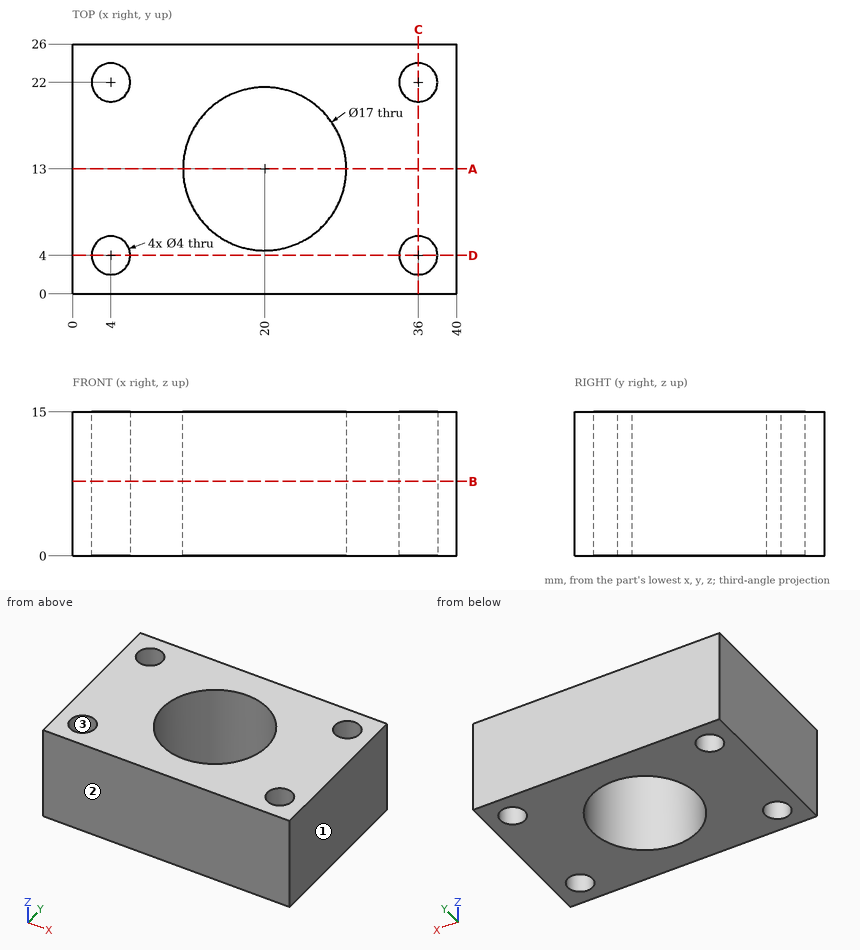
For this review, use the dimensioned drawing (mm, ordinates from the lowest corner) and the shaded views. Give positions to 0.01 mm unless a question says otherwise; leave off trailing zeros. Order: outer loops, then holes, each group sorted by start corner. A loop starts at its lowest first (then second) coordinate and runs counter-clockwise, first axis right, second up. Notation, with made-up numbers: (13.5, 28) - (58.5, 28) arc R21 cw to (58.5, 37) - close; hole circle Ø9 at (26.5, -28.5). An arc over 180 degrees is marked (long way). Write item = value, one per line. Start each with the question number.
Q1. We need section B-B on z = 7.75. State the section outline as (x, y) points, plus the area to 3 significant figures.
Q2. Mouldability with a two-part tool opening along X and no side actions: class the marked faces 1, 2 and 3 as released by +X, released by -X, zero draft, split by the parting line, or undercut.
Q3. We need section C-C on x = 36. State the section outline as (y, z) points.
Q4. To check wall thickness, follow L1, parallel to Y at x = 4, z = 5.25; L2, parallel to X at y = 2.25, z = 14.25; L3, parallel to Y at x = 37.5, z = 10.5. State the ranges of each line that lie inside material, in increasing order. Write a range as from..to.
Q5. We need section A-A on y = 13. State the section outline as (x, z) points.
Q6. Clearance check with a flat-ended pin moving along its axis: pin 1 Ø3 at (x, y) = (36, 4) entering from -Z. State where the tip first meets the part, or that it passes through.
Q7. We need section D-D on y = 4. State the section outline as (x, z) points, plus the area to 3 significant figures.
Working result:
q1.outline = (0, 0) - (40, 0) - (40, 26) - (0, 26) - close; hole circle Ø4 at (4, 4); hole circle Ø4 at (4, 22); hole circle Ø17 at (20, 13); hole circle Ø4 at (36, 4); hole circle Ø4 at (36, 22)
q1.area = 763 mm²
q2.face_1 = released by +X
q2.face_2 = zero draft
q2.face_3 = undercut
q3.outline = (0, 0) - (2, 0) - (2, 15) - (0, 15) - close; (6, 0) - (20, 0) - (20, 15) - (6, 15) - close; (24, 0) - (26, 0) - (26, 15) - (24, 15) - close
q4.L1 = 0..2, 6..20, 24..26
q4.L2 = 0..3.03, 4.97..35.03, 36.97..40
q4.L3 = 0..2.68, 5.32..20.68, 23.32..26
q5.outline = (0, 0) - (11.5, 0) - (11.5, 15) - (0, 15) - close; (28.5, 0) - (40, 0) - (40, 15) - (28.5, 15) - close
q6.pin_1 = through
q7.outline = (0, 0) - (2, 0) - (2, 15) - (0, 15) - close; (6, 0) - (34, 0) - (34, 15) - (6, 15) - close; (38, 0) - (40, 0) - (40, 15) - (38, 15) - close
q7.area = 480 mm²
